Can you work these out from the model? Positions are in its coordinate system, mm. Face numbers are marked on the shaded views. A direction names the side the tool comes from. Give positions to 0.01 mm unless a question says otherwise; leave off trailing zeros. Loops run counter-clockwise (first coordinate to the right, second up) from the corner with the lowest first, then second, coordinate; pieces in that order, holes last.
Autodesk Fusion 360 part; units mm, degrees
sketch "Sketch1" plane through (0, 0, 0) normal (0, 0, 1) x (1, 0, 0)
  circle A0 centre (0, 0) radius 17.25
  circle A1 centre (0, 0) radius 19.25
  line L0 (0, 19.25) -> (5, 19.25) construction
  line L1 (5, 19.25) -> (-5, 19.25) construction
  line L2 (-5, 19.25) -> (-5, 22.75) construction
  line L3 (-5, 22.75) -> (5, 22.75) construction
  line L4 (5, 22.75) -> (5, 19.25) construction
  line L5 (-5, 22.75) -> (-5, 18.5893)
  line L6 (-5, 22.75) -> (5, 22.75)
  line L7 (5, 18.5893) -> (5, 22.75)
  line L8 (0, 0) -> (17.25, 0) construction
  line L9 (-5, -22.75) -> (-5, -18.5893)
  line L10 (-5, -22.75) -> (5, -22.75)
  line L11 (5, -18.5893) -> (5, -22.75)
  circle A2 centre (0, 0) radius 1.5
  circle A3 centre (0, 0) radius 35
  line L12 (-19.2494, 0.1529) -> (-34.9997, 0.1529) construction
  circle A4 centre (-27.1245, 0.1529) radius 1.5
  circle A5 centre (-8.5273, -25.7497) radius 1.5
  circle A6 centre (21.8543, -16.0671) radius 1.5
  circle A7 centre (22.0341, 15.8197) radius 1.5
  circle A8 centre (-8.2366, 25.8442) radius 1.5
  line L13 (-34.9997, 0.1529) -> (-36, 0.1529) construction
  line L14 (-36, 0.1529) -> (-36, 32.1529) construction
  line L15 (-36, 32.1529) -> (-64, 32.1529)
  line L16 (-64, 32.1529) -> (-64, -31.8471)
  line L17 (-64, -31.8471) -> (-36, -31.8471)
  line L18 (-36, -31.8471) -> (-36, 32.1529)
  line L19 (-65, 33.1529) -> (-65, -32.8471)
  line L20 (-65, -32.8471) -> (-35, -32.8471)
  line L21 (-35, -32.8471) -> (-35, 33.1529)
  line L22 (-35, 33.1529) -> (-65, 33.1529)
  line L23 (0, -35) -> (-35, -32.8471)
  line L24 (0, 35) -> (-35, 33.1529)
  dimension "d1" = 34.5
  dimension "d2" = 2
  dimension "d3" = 5
  dimension "d4" = 10
  dimension "d5" = 3.5
  dimension "d6" = 3
  dimension "d17" = 70
  dimension "d18" = 3
  dimension "d20" = 360
  dimension "d24" = 32
  dimension "d25" = 28
  dimension "d26" = 64
  dimension "d27" = 1
extrude "Extrude1" add sketch "Sketch1" along normal blind 9 contours A1
extrude "Extrude2" add sketch "Sketch1" along normal blind 2 contours A0 | A3 L23 L24 | A3 L24 | A3 L23 | A3 L21 L24 | A3 L21 L23
extrude "Extrude3" add sketch "Sketch1" against normal blind 1.5 from surface at 9 contours A1 L5 L6 L7 | A1 L9 L10 L11
chamfer "Chamfer1" distance 0.25 angle 45 4 edges at (-5, 20.6697, 9) (5, 20.6697, 9) (5, -20.6697, 9) (-5, -20.6697, 9)
chamfer "Chamfer2" distance 0.25 angle 45 4 edges at (5, -20.6697, 7.5) (-5, -20.6697, 7.5) (-5, 20.6697, 7.5) (5, 20.6697, 7.5)
chamfer "Chamfer4" distance 1.5 angle 45 5 edges at (-28.523, 0.6953, 2) (20.6356, 16.3621, 2) (20.4559, -15.5247, 2) (-9.9258, -25.2073, 2) (-9.635, 26.3866, 2)
fillet "Fillet1" radius 1 4 edges at (5, 22.75, 8.25) (-5, 22.75, 8.25) (-5, -22.75, 8.25) (5, -22.75, 8.25)
extrude "Extrude4" add sketch "Sketch1" along normal blind 4 contours L19 L20 L21 L22
sketch "Sketch2" plane through (0, -32.8471, 0) normal (0, -1, 0) x (1, 0, 0)
  line L0 (-65, 0) -> (-35, 0)
  line L1 (-35, 0) -> (-35, 2)
  line L2 (-35, 2) -> (-35, 4)
  line L3 (-35, 4) -> (-65, 4)
  line L4 (-65, 4) -> (-65, 0)
  line L5 (-35, 4) -> (-35, 0) construction
  line L6 (-36, 3.5) -> (-37.3, 4)
  line L7 (-37.3, 4) -> (-36, 4)
  line L8 (-36, 3.5) -> (-36, 4)
  line L9 (-64, 3.5) -> (-62.7, 4)
  line L10 (-62.7, 4) -> (-64, 4)
  line L11 (-64, 3.5) -> (-64, 4)
extrude "Extrude5" add sketch "Sketch2" against normal blind 7 from surface at -27 contours L3 L9 L10 L11
extrude "Extrude6" add sketch "Sketch2" against normal blind 5 from surface at -23 contours L3 L6 L7 L8
extrude "Extrude8" add sketch "Sketch1" along normal blind 0.2 contours L15 L16 L17 L18
extrude "Extrude9" add sketch "Sketch2" against normal blind 5 from surface at -50 contours L3 L6 L7 L8
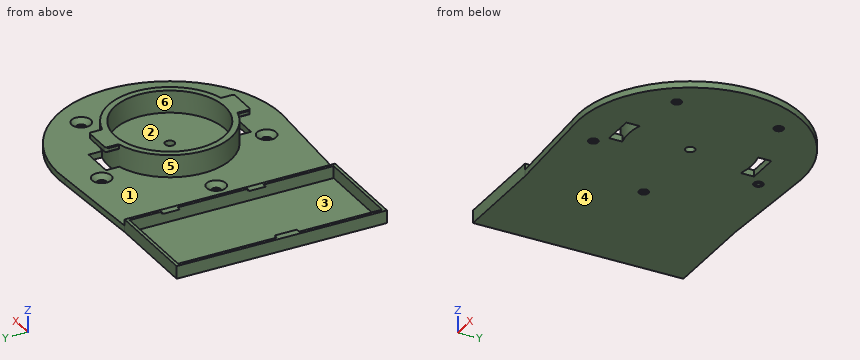
(1) Thinking about a two-plate mould opening in Y: for the marked faces 1, 2 and 3, which applies, pulls with the +Y half, pulls with the -Y half, needs draft (parallel to the pull), parting line crosses it, or undercut?
Returned:
face 1: needs draft
face 2: undercut
face 3: undercut
(2) Suppose I cut it at C-C on x = -14.5. List the corners of the cut face in (y, z) for me.
Returned:
outline: (-34.11, 0) - (34.23, 0) - (34.23, 2) - (12.66, 2) - (12.66, 9) - (9.34, 9) - (9.34, 2) - (-9.34, 2) - (-9.34, 9) - (-12.66, 9) - (-12.66, 2) - (-34.11, 2) - close
(3) Please list where these lines run through material, in increasing order: probe 1 along Y at (x, z) = (0, 0.8); probe 2 along X at (y, z) = (26.5, 3); probe 3 along Z at (x, y) = (-8.5, 30).
Returned:
probe 1: y = -35 to -22.75, -19.25 to -1.5, 1.5 to 19.25, 22.75 to 35
probe 2: x = -65 to -64, -36 to -35
probe 3: z = 0 to 2
(4) Will these pins go through, and if not, where does the flat tip stop? P1, Ø2, axis at x = -8.5, z = 7.5, coming from the +Y side; P2, Ø0.6, axis at x = -36.5, z = 3.5, coming from the -Y side; P3, Ø1.6, axis at x = 1.5, z = 8.5, coming from the -Y side.
Returned:
P1: stops at y = 17.73
P2: stops at y = -32.85
P3: stops at y = -22.75
(5) Suppose I cut it at B-B on x = -49.5. List the corners of the cut face in (y, z) for me, plus the area to 3 significant figures.
Returned:
outline: (-32.85, 0) - (33.15, 0) - (33.15, 4) - (32.15, 4) - (32.15, 0.2) - (-31.85, 0.2) - (-31.85, 4) - (-32.85, 4) - close
area: 20.8 mm2
(6) Suppose I cut it at A-A on x = 0. List the corners of the cut face in (y, z) for me, plus the area to 4 significant figures.
Returned:
outline: (-35, 0) - (-22.75, 0) - (-22.75, 2) - (-35, 2) - close; (-22.75, 7.5) - (-19.25, 7.5) - (-19.25, 0) - (-1.5, 0) - (-1.5, 2) - (-17.25, 2) - (-17.25, 9) - (-22.75, 9) - close; (1.5, 0) - (19.25, 0) - (19.25, 7.5) - (22.75, 7.5) - (22.75, 9) - (17.25, 9) - (17.25, 2) - (1.5, 2) - close; (22.75, 0) - (35, 0) - (35, 2) - (22.75, 2) - close
area: 158.5 mm2
(7) Which directions (+Z, -Z, +X, -X, +Y, -Y) give clear straight access to the entire face, cutting with the end or side of a thin tool? Please do the marked faces 4, 5 and 6.
Returned:
face 4: -Z, +X, -X, +Y, -Y
face 5: none
face 6: +Z
(8) Suppose I cut it at D-D on x = 11.5. List the corners of the cut face in (y, z) for me.
Returned:
outline: (-33.06, 0) - (33.06, 0) - (33.06, 2) - (15.44, 2) - (15.44, 9) - (12.86, 9) - (12.86, 2) - (-12.86, 2) - (-12.86, 9) - (-15.44, 9) - (-15.44, 2) - (-33.06, 2) - close
